Verification items for this drawing (mm, ordinates from the low corner). Round coordinates to 2 decimals unless told otherwise and drop trailing zeros. Order: outer loops, then holes, each group sorted by start corner. A loop starts at its lowest first (then second) coordinate and runs counter-clockwise, first axis right, second up. Notation, with made-up numbers: (42.5, -11) -> (55.5, -11) arc R29 ccw to (55.5, 18) -> close; hole circle Ø5 at (76.25, -30). An arc over 180 degrees is marked (long way). Return JSON: item names as keys, results as strings. Group by question number.
Item 1: Sectioned sample at C-C on y = 0.5. Record the cut outline in (x, z).
Item 2: Scan lines: probe 1 along Z at (x, y) = (37.5, 1.05); probe 2 along Z at (x, y) = (19.5, 2.95). Record each from-to range of solid material in increasing order. Write a range as from..to.
Item 3: Sectioned sample at B-B on x = 10. Record the cut outline in (y, z).
Item 4: Depth check by flat-ended pin: pin 1 Ø2.5 at (x, z) = (60, 5) entering from -Y. Enter the tip coordinate at first touch or a pass-through.
Item 5: Sectioned sample at D-D on x = 40. Record the cut outline in (y, z).
Item 6: Sectioned sample at A-A on z = 5. Record the cut outline in (x, y).
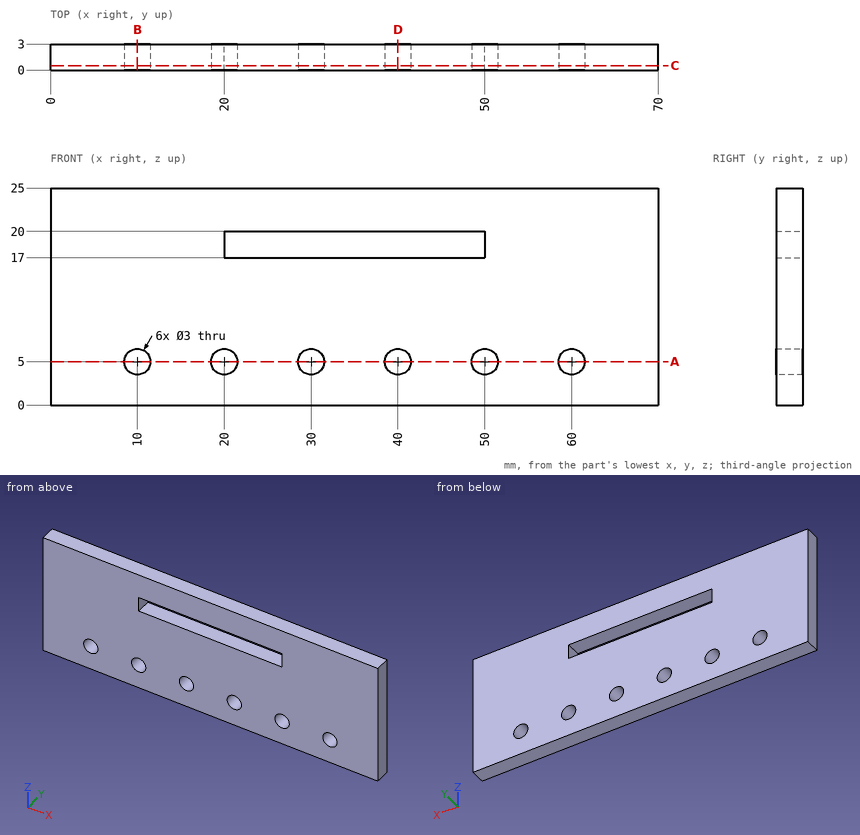
Recorded:
{
 "1": {"outline": "(0, 0) -> (70, 0) -> (70, 25) -> (0, 25) -> close; hole circle Ø3 at (10, 5); hole circle Ø3 at (20, 5); hole (20, 17) -> (50, 17) -> (50, 20) -> (20, 20) -> close; hole circle Ø3 at (30, 5); hole circle Ø3 at (40, 5); hole circle Ø3 at (50, 5); hole circle Ø3 at (60, 5)"},
 "2": {"probe 1": "0..17, 20..25", "probe 2": "0..3.59, 6.41..25"},
 "3": {"outline": "(0, 0) -> (3, 0) -> (3, 3.5) -> (0, 3.5) -> close; (0, 6.5) -> (3, 6.5) -> (3, 25) -> (0, 25) -> close"},
 "4": {"pin 1": "through"},
 "5": {"outline": "(0, 0) -> (3, 0) -> (3, 3.5) -> (0, 3.5) -> close; (0, 6.5) -> (3, 6.5) -> (3, 17) -> (0, 17) -> close; (0, 20) -> (3, 20) -> (3, 25) -> (0, 25) -> close"},
 "6": {"outline": "(0, 0) -> (8.5, 0) -> (8.5, 3) -> (0, 3) -> close; (11.5, 0) -> (18.5, 0) -> (18.5, 3) -> (11.5, 3) -> close; (21.5, 0) -> (28.5, 0) -> (28.5, 3) -> (21.5, 3) -> close; (31.5, 0) -> (38.5, 0) -> (38.5, 3) -> (31.5, 3) -> close; (41.5, 0) -> (48.5, 0) -> (48.5, 3) -> (41.5, 3) -> close; (51.5, 0) -> (58.5, 0) -> (58.5, 3) -> (51.5, 3) -> close; (61.5, 0) -> (70, 0) -> (70, 3) -> (61.5, 3) -> close"}
}
